from build123d import *

# Parameters (mm, degrees)
SCHIZZO1_R                   = 50
ESTRUSIONE_ESTRUSIONE1_DEPTH = 30
SCHIZZO2_R                   = 10
ESTRUSIONE_ESTRUSIONE2_DEPTH = 5
ESTRUSIONE_ESTRUSIONE3_START = 5
SCHIZZO3_R                   = 10
ESTRUSIONE_ESTRUSIONE3_DEPTH = 5
SCHIZZO4_R                   = 10
ESTRUSIONE_ESTRUSIONE4_DEPTH = 5
ESTRUSIONE_ESTRUSIONE5_START = 5
SCHIZZO5_R                   = 10
ESTRUSIONE_ESTRUSIONE5_DEPTH = 5
SCHIZZO6_W                   = 105
SCHIZZO6_H                   = 80
ESTRUSIONE_ESTRUSIONE6_DEPTH = 2
SCHIZZO7_R                   = 2.5
TAGLIO_ESTRUSIONE1_DEPTH     = 2


with BuildPart() as part:
    # Schizzo1 → Estrusione-Estrusione1 (new body)
    with BuildSketch(Plane.XY):
        Circle(SCHIZZO1_R)
    extrude(amount=ESTRUSIONE_ESTRUSIONE1_DEPTH)

    # Schizzo2 → Estrusione-Estrusione2 (add)
    with BuildSketch(Plane.XY.offset(30)):
        Circle(SCHIZZO2_R)
    extrude(amount=ESTRUSIONE_ESTRUSIONE2_DEPTH)

    # Schizzo3 → Estrusione-Estrusione3 (add)
    with BuildSketch(Plane(origin=(0, 0, 0), x_dir=(-1, 0, 0), z_dir=(0, 0, -1)).offset(ESTRUSIONE_ESTRUSIONE3_START)):
        with Locations(Location((0, 0, 0), (0, 0, 180))):
            Circle(SCHIZZO3_R)
    extrude(amount=-ESTRUSIONE_ESTRUSIONE3_DEPTH)

    # Schizzo4 → Estrusione-Estrusione4 (add)
    with BuildSketch(Plane.XY.offset(35)):
        with Locations(Location((0, 0, 0), (0, 0, 116.565051177))):
            Circle(SCHIZZO4_R)
        Polygon((0, 80), (-40, 80), (0, 0), align=None)
        with BuildLine():
            Line((-4.472135955, 8.94427191), (0, 0))
            Line((0, 0), (0, 10))
            ThreePointArc((0, 10), (-2.297529205, 9.732489895), (-4.472135955, 8.94427191))
        make_face()
        with BuildLine():
            Line((0, 10), (0, 0))
            Line((0, 0), (-4.472135955, 8.94427191))
            ThreePointArc((-4.472135955, 8.94427191), (-5.257311121, -8.506508084), (10, 0))
            ThreePointArc((10, 0), (7.071067812, 7.071067812), (0, 10))
        make_face()
    extrude(amount=ESTRUSIONE_ESTRUSIONE4_DEPTH)

    # Schizzo5 → Estrusione-Estrusione5 (add)
    with BuildSketch(Plane(origin=(0, 0, -5), x_dir=(-1, 0, 0), z_dir=(0, 0, -1)).offset(ESTRUSIONE_ESTRUSIONE5_START)):
        with Locations(Location((0, 0, 0), (0, 0, 63.434948823))):
            Circle(SCHIZZO5_R)
        Polygon((40, 80), (0, 0), (0, 80), align=None)
        with BuildLine():
            Line((4.472135955, 8.94427191), (0, 0))
            Line((0, 0), (0, 10))
            ThreePointArc((0, 10), (-7.071067812, -7.071067812), (10, 0))
            ThreePointArc((10, 0), (8.506508084, 5.257311121), (4.472135955, 8.94427191))
        make_face()
        with BuildLine():
            Line((0, 10), (0, 0))
            Line((0, 0), (4.472135955, 8.94427191))
            ThreePointArc((4.472135955, 8.94427191), (2.297529205, 9.732489895), (0, 10))
        make_face()
    extrude(amount=-ESTRUSIONE_ESTRUSIONE5_DEPTH)

    # Schizzo6 → Estrusione-Estrusione6 (add)
    with BuildSketch(Plane(origin=(0, 80, 0), x_dir=(1, 0, 0), z_dir=(0, 1, 0))):
        with Locations((-40, -15)):
            Rectangle(SCHIZZO6_W, SCHIZZO6_H)
    extrude(amount=-ESTRUSIONE_ESTRUSIONE6_DEPTH)

    # Schizzo7 → Taglio-Estrusione1 (cut)
    with BuildSketch(Plane(origin=(0, 80, 0), x_dir=(1, 0, 0), z_dir=(0, 1, 0))):
        with Locations(Location((-77.5, -40, 0), (0, 0, 270))):
            Circle(SCHIZZO7_R)
        with Locations(Location((-2.5, -40, 0), (0, 0, 180))):
            Circle(SCHIZZO7_R)
        with Locations(Location((-2.5, 10, 0), (0, 0, 270))):
            Circle(SCHIZZO7_R)
        with Locations(Location((-77.5, 10, 0), (0, 0, 90))):
            Circle(SCHIZZO7_R)
    extrude(amount=-TAGLIO_ESTRUSIONE1_DEPTH, mode=Mode.SUBTRACT)


solid = part.part
Here's how the part is built. I have some questions about the finished solid (model axes, mm). A direction names the side the tool comes from. Give positions to 0.01 mm unless a question says otherwise; leave off trailing zeros. Loops run counter-clockwise (first coordinate to the right, second up) from the corner with the lowest first, then second, coordinate; pieces in that order, holes last. Notation, with made-up numbers: (77.5, 74.25) -> (92.5, 74.25) arc R18 ccw to (92.5, 86.25) -> close; hole circle Ø3 at (34, 64). An arc over 180 degrees is marked (long way). Answer as a JSON object with one key per item and string values. Group by question number.
Item 1: Imagine slicing it at D-D on x = -2.5. Write out the boundary of the cut face in (y, z), then the cut area to 3 significant figures.
Item 2: Imagine slicing it at A-A on z = 25.5. Write out the boundary of the cut face in (x, y), then the cut area to 3 significant figures.
Item 3: Imagine slicing it at C-C on y = 15.5. Write out the boundary of the cut face in (x, z), then the cut area to 3 significant figures.
Item 4: I need wall thicknesses on L1, parallel to Z at x = -2.5, y = 79.25; L2, parallel to X at y = 79, z = -10; L3, parallel to Y at x = 0, z = 34. Which ranges of each line are inside material? Lowest first, please.
Item 5: Thinking about a two-plate mould opening in Y: for faces 6 (the flat face through (-41, 80, 14)), 7 (the flat face through (-11, 37, 40)), 8 (the cylindrical face through (8.817, 4.718, -5.07)), which applies, pulls with the +Y half, pulls with the -Y half, needs draft (parallel to the pull), parting line crosses it, or undercut?
Item 6: Will these pins go through, and if not, where does the flat tip stop? pin 1 (4 mm diameter, centred on x = -77.5, z = -10, fed in from -Y); pin 2 (3 mm diameter, centred on x = -1.5, z = -8.5, fed in from +Y); pin 3 (5.5 mm diameter, centred on y = 52, z = 38.5, fed in from +X); pin 4 (6 mm diameter, centred on x = -8.5, z = 12, fed in from -Y).
Item 7: On a 3-axis mill with a long thin cutter (end or side, diameter ignored), from which of +Z, -Z, +X, -X, +Y, -Y can I reach the whole of each face in a straight line? I mean faces 1 (the flat face through (-17, 55, 35)), 2 (the flat face through (0, 44, 37)), 3 (the flat face through (-10, 37, -10)), 4 (the cylindrical face through (-75.28, 79.01, -11.15)), 5 (the cylindrical face through (-2.4, 79, -12.5)). Say none if no direction works.
Item 8: Imagine slicing it at B-B on x = -77.5. Write out the boundary of the cut face in (y, z), then the cut area to 3 significant figures.
Answer list:
{
 "1": {"outline": "(-49.94, 0) -> (-9.68, 0) -> (-9.68, -10) -> (78, -10) -> (78, -7.5) -> (80, -7.5) -> (80, 37.5) -> (78, 37.5) -> (78, 40) -> (-9.68, 40) -> (-9.68, 30) -> (-49.94, 30) -> close; (78, -25) -> (80, -25) -> (80, -12.5) -> (78, -12.5) -> close; (78, 42.5) -> (80, 42.5) -> (80, 55) -> (78, 55) -> close; hole (9.68, -5) -> (78, -5) -> (78, 35) -> (9.68, 35) -> (9.68, 30) -> (49.94, 30) -> (49.94, 0) -> (9.68, 0) -> close", "area": "4,210 mm2"},
 "2": {"outline": "(-92.5, 78) -> (12.5, 78) -> (12.5, 80) -> (-92.5, 80) -> close; circle Ø100 at (0, 0)", "area": "8,060 mm2"},
 "3": {"outline": "(-47.54, 0) -> (47.54, 0) -> (47.54, 30) -> (-47.54, 30) -> close; (-7.75, -10) -> (0, -10) -> (0, -5) -> (-7.75, -5) -> close; (-7.75, 35) -> (0, 35) -> (0, 40) -> (-7.75, 40) -> close", "area": "2,930 mm2"},
 "4": {"L1": "z = -25 to -12.5, -7.5 to 37.5, 42.5 to 55", "L2": "x = -92.5 to -80, -75 to -5, 0 to 12.5", "L3": "y = -10 to 10, 78 to 80"},
 "5": {"face 6": "pulls with the +Y half", "face 7": "needs draft", "face 8": "undercut"},
 "6": {"pin 1": "passes through", "pin 2": "stops at y = 80", "pin 3": "stops at x = 0", "pin 4": "stops at y = -49.7"},
 "7": {"face 1": "+X, -X", "face 2": "+Z, +X", "face 3": "-Z, +X, -X, -Y", "face 4": "+Y, -Y", "face 5": "+Y"},
 "8": {"outline": "(78, -25) -> (80, -25) -> (80, -12.5) -> (78, -12.5) -> close; (78, -7.5) -> (80, -7.5) -> (80, 37.5) -> (78, 37.5) -> close; (78, 42.5) -> (80, 42.5) -> (80, 55) -> (78, 55) -> close", "area": "140 mm2"}
}
